Input: part model. Units: mm. Frame: model coordinates. A direction names the side the tool comes from. Round coordinates to 2 decimals unless told otherwise and drop trailing zeros. Order: outer loops, then holes, each group sorted by start corner. A loop starts at its lowest first (then second) coordinate and runs counter-clockwise, first axis right, second up. Notation, with made-up numbers: (38.5, 83.25) -> (79.5, 83.25) arc R17 cw to (79.5, 103.25) -> close; hole circle Ø10 at (-1.5, 40.5). An arc over 180 degrees is marked (long way). Use a Markdown table: item, result.
from build123d import *
from build123d.topology import SkipClean

# Parameters (mm, degrees)
SKETCH1_W                = 11.772507028
SKETCH1_H                = 7.5
SKETCH1_R                = 1
SKETCH1_R_2              = 3
SKETCH1_R_3              = 1.35
BOSS_EXTRUDE1_DEPTH      = 3
SKETCH4_W                = 1.65
SKETCH4_H                = 4.12
CHAMFER1_SIZE            = 0.5
CHAMFER1_OF_MIRROR1_SIZE = 0.5


with BuildPart() as part:
    # Sketch1 → Boss-Extrude1 (new body)
    # profile 1 of 5: a face of its own
    with BuildSketch(Plane(origin=(0, 0, 0), x_dir=(1, 0, 0), z_dir=(0, 1, 0))):
        with BuildLine():
            Line((5.886253514, 0), (5.886253514, -7.5))
            ThreePointArc((5.886253514, -7.5), (10.206881736, -9.07831948), (12.492796705, -13.07))
            ThreePointArc((12.492796705, -13.07), (15.492796705, -10.07), (18.492796705, -13.07))
            ThreePointArc((18.492796705, -13.07), (14.965761089, -3.857208203), (5.886253514, 0))
        make_face()
    # profile 2 of 5: a face of its own
    with BuildSketch(Plane(origin=(0, 0, 0), x_dir=(1, 0, 0), z_dir=(0, 1, 0))):
        with Locations((0, -3.75)):
            Rectangle(SKETCH1_W, SKETCH1_H)
        with Locations(Location((0, -2.1, 0), (0, 0, 270))):
            Circle(SKETCH1_R, mode=Mode.SUBTRACT)
        with Locations(Location((4.75, -4.7, 0), (0, 0, 270))):
            Circle(SKETCH1_R, mode=Mode.SUBTRACT)
        with Locations(Location((-4.75, -4.7, 0), (0, 0, 270))):
            Circle(SKETCH1_R, mode=Mode.SUBTRACT)
    # profile 3 of 5: a face of its own
    with BuildSketch(Plane(origin=(0, 0, 0), x_dir=(1, 0, 0), z_dir=(0, 1, 0))):
        with BuildLine():
            ThreePointArc((-12.492796705, -13.07), (-10.206881736, -9.07831948), (-5.886253514, -7.5))
            Line((-5.886253514, -7.5), (-5.886253514, 0))
            ThreePointArc((-5.886253514, 0), (-14.965761089, -3.857208203), (-18.492796705, -13.07))
            ThreePointArc((-18.492796705, -13.07), (-15.492796705, -10.07), (-12.492796705, -13.07))
        make_face()
    # profile 4 of 5: a face of its own
    with BuildSketch(Plane(origin=(0, 0, 0), x_dir=(1, 0, 0), z_dir=(0, 1, 0))):
        with Locations((-15.492796705, -13.07)):
            Circle(SKETCH1_R_2)
        with Locations(Location((-15.492796705, -13.07, 0), (0, 0, 270))):
            Circle(SKETCH1_R_3, mode=Mode.SUBTRACT)
    # profile 5 of 5: a face of its own
    with BuildSketch(Plane(origin=(0, 0, 0), x_dir=(1, 0, 0), z_dir=(0, 1, 0))):
        with Locations((15.492796705, -13.07)):
            Circle(SKETCH1_R_2)
        with Locations(Location((15.492796705, -13.07, 0), (0, 0, 270))):
            Circle(SKETCH1_R_3, mode=Mode.SUBTRACT)
    extrude(amount=BOSS_EXTRUDE1_DEPTH)

    # Sketch4 → Revolve2 (revolve)
    with BuildSketch(Plane.XY.offset(13.07), mode=Mode.PRIVATE) as revolve2_sk:
        with Locations((-17.667796705, 5.06)):
            Rectangle(SKETCH4_W, SKETCH4_H)
    revolve2 = revolve(revolve2_sk.sketch.rotate(Axis((-15.492796705, 3, 13.07), (0, -1, 0)), 180), axis=Axis((-15.492796705, 3, 13.07), (0, -1, 0)))

    # Chamfer1
    chamfer1_edges = [part.edges().sort_by_distance(p)[0] for p in [
        (-16.842796705, 7.12, 13.07),
    ]]
    chamfer(chamfer1_edges, length=CHAMFER1_SIZE)

    # Mirror1: Revolve2 across plane
    with SkipClean():  # the faces are left unmerged after this step: merging them gives an invalid solid
        add(revolve2.mirror(Plane(origin=(0, 0, 0), x_dir=(0, 0, 1), z_dir=(1, 0, 0))))

    # Chamfer1 of Mirror1
    chamfer1_of_mirror1_edges = [part.edges().sort_by_distance(p)[0] for p in [
        (16.842796705, 7.12, 13.07),
    ]]
    chamfer(chamfer1_of_mirror1_edges, length=CHAMFER1_OF_MIRROR1_SIZE)


solid = part.part
1) Ray query, probe 1 along X at (y, z) = (2.05, 13.07); probe 2 along X at (y, z) = (1.5, 14.25); probe 3 along X at (y, z) = (2, 4.7). Return the intervals inside material, ascending.
Answer key:
| item | result |
|---|---|
| probe 1 | x = -18.49 to -16.84, -14.14 to -12.49, 12.49 to 14.14, 16.84 to 18.49 |
| probe 2 | x = -18.25 to -16.15, -14.84 to -12.73, 12.73 to 14.84, 16.15 to 18.25 |
| probe 3 | x = -15.71 to -5.75, -3.75 to 3.75, 5.75 to 15.71 |
2) Cut plane D-D on z = 4.7. Return loops of the section in (x, y), and give its area (3 significant figures).
Answer key:
| item | result |
|---|---|
| outline | (-15.71, 0) -> (-5.75, 0) -> (-5.75, 3) -> (-15.71, 3) -> close; (-3.75, 0) -> (3.75, 0) -> (3.75, 3) -> (-3.75, 3) -> close; (5.75, 0) -> (15.71, 0) -> (15.71, 3) -> (5.75, 3) -> close |
| area | 82.3 mm^2 |
3) Set-up query: faces 5 (the face through (0, 0, 6)), 6 (the face through (0, 1, 7.5)), 7 (the face through (-15.883, 4.401, 16.044)). Return all of +Z, -Z, +X, -X, +Y, -Y with unobstructed straight access to the full face (end or side cutting, diameter ignored); none if empty.
Answer key:
| item | result |
|---|---|
| face 5 | +Z, -Z, +X, -X, -Y |
| face 6 | +Z, +Y, -Y |
| face 7 | +Y |
4) Cut plane C-C on z = 2.1. Return loops of the section in (x, y).
Answer key:
| item | result |
|---|---|
| outline | (-12.86, 0) -> (-1, 0) -> (-1, 3) -> (-12.86, 3) -> close; (1, 0) -> (12.86, 0) -> (12.86, 3) -> (1, 3) -> close |
5) Cut plane A-A on x = 0. Return loops of the section in (y, z), and give its area (3 significant figures).
Answer key:
| item | result |
|---|---|
| outline | (0, 0) -> (3, 0) -> (3, 1.1) -> (0, 1.1) -> close; (0, 3.1) -> (3, 3.1) -> (3, 7.5) -> (0, 7.5) -> close |
| area | 16.5 mm^2 |
6) Contact query for flat-ended pins moving along their axis: P1, Ø3.5, axis at x = 15.49, z = 13.07, coming from the +Y side; P2, Ø1.5, axis at x = 0.5, y = 1, coming from the +Z side; P3, Ø6, axis at x = -1.5, z = 9.5, coming from the +Y side; P4, Ø1.6, axis at x = 0, z = 2.1, coming from the -Y side. Output: stop coordinate, or through.
Answer key:
| item | result |
|---|---|
| P1 | stops at y = 7.02 |
| P2 | stops at z = 7.5 |
| P3 | stops at y = 3 |
| P4 | passes through |
7) Cut plane B-B on y = 4. Return loops of the section in (x, z), and give its area (3 significant figures).
Answer key:
| item | result |
|---|---|
| outline | circle Ø6 at (-15.49, 13.07); circle Ø6 at (15.49, 13.07); hole circle Ø2.7 at (-15.49, 13.07); hole circle Ø2.7 at (15.49, 13.07) |
| area | 45.1 mm^2 |
8) Draft query along Z for faces 1 (the face through (-4.074, 1.479, 3.963)), 2 (the face through (0, 1, 0)), 3 (the face through (10.16, 1.48, 9.04)), 4 (the face through (-14.24, 3.36, 13.57)). Return one class per face: released by +Z, released by -Z, zero draft, split by the parting line, or undercut.
Answer key:
| item | result |
|---|---|
| face 1 | undercut |
| face 2 | released by -Z |
| face 3 | released by +Z |
| face 4 | undercut |
